from build123d import *

# Parameters (mm, degrees)
SKETCH_1_R      = 11
EXTRUDE_1_DEPTH = 7
SKETCH_2_R      = 6
EXTRUDE_2_DEPTH = 3
FILLET_1_R      = 2
THREAD_1_PITCH  = 1
SKETCH_9_W      = 0.25
SKETCH_9_H      = 0.05


with BuildPart() as part:
    # Sketch 1 → 凸台-拉伸1 (new body)
    with BuildSketch(Plane(origin=(0, 0, 0), x_dir=(1, 0, 0), z_dir=(0, 1, 0))):
        with Locations(Location((0, 0, 0), (0, 0, 270))):
            Circle(SKETCH_1_R)
    extrude(amount=EXTRUDE_1_DEPTH)

    # 草图2 → 凸台-拉伸2 (add)
    with BuildSketch(Plane(origin=(0, 7, 0), x_dir=(1, 0, 0), z_dir=(0, 1, 0))):
        with Locations(Location((0, 0, 0), (0, 0, 270))):
            Circle(SKETCH_2_R)
    extrude(amount=EXTRUDE_2_DEPTH)

    # 圆角1
    fillet_1_edges = [part.edges().sort_by_distance(p)[0] for p in [
        (0, 0, -11),
    ]]
    fillet(fillet_1_edges, radius=FILLET_1_R)

    # 螺纹线1: the profile of Sketch 1 2 profile screwed along a right-hand helix of 3 turns, 8 arcs to a turn; built about Z, then put on its axis
    thread_1_z = Axis((0, 0, 0), (0, 0, 1))
    thread_1_corners = [(5.9997, 0, -0.000173205), (6.541265875, 0, 0.312499999), (6.541265875, 0, 0.437499999), (5.9997, 0, 0.750173202)]
    with BuildLine(mode=Mode.PRIVATE) as thread_1_profile:
        Line(thread_1_corners[0], thread_1_corners[1])
        Line(thread_1_corners[1], thread_1_corners[2])
        Line(thread_1_corners[2], thread_1_corners[3])
        Line(thread_1_corners[3], thread_1_corners[0])
    thread_1_cap = Face(thread_1_profile.wire())
    thread_1_turn_angles = [0, 22.5, 45, 67.5, 90, 112.5, 135, 157.5, 180, 202.5, 225, 247.5, 270, 292.5, 315, 337.5, 360]
    thread_1_turn_weights = [1, 0.9238795325112867, 1, 0.9238795325112867, 1, 0.9238795325112867, 1, 0.9238795325112867, 1, 0.9238795325112867, 1, 0.9238795325112867, 1, 0.9238795325112867, 1, 0.9238795325112867, 1]
    thread_1_turn_rails = [Edge.make_bspline([Vector(p[0], p[1], 0).rotate(thread_1_z, thread_1_turn_angles[k]) / thread_1_turn_weights[k] + Vector(0, 0, p[2] + THREAD_1_PITCH * thread_1_turn_angles[k] / 360) for k in range(17)], [0, 0, 0, 1, 1, 2, 2, 3, 3, 4, 4, 5, 5, 6, 6, 7, 7, 8, 8, 8], 2, thread_1_turn_weights) for p in thread_1_corners]
    thread_1_turn_sides = [Face.make_surface_from_curves(thread_1_turn_rails[p[0]], thread_1_turn_rails[p[1]]) for p in [(0, 1), (1, 2), (2, 3), (3, 0)]]
    thread_1 = Plane(origin=(0, 10, 0), x_dir=(-1, 0, 0), z_dir=(0, -1, 0)) * Solid(Shell([*[p.moved(Location((0, 0, THREAD_1_PITCH * i))) for i in range(3) for p in thread_1_turn_sides], thread_1_cap, thread_1_cap.rotate(thread_1_z, 1080).moved(Location((0, 0, THREAD_1_PITCH * 1080 / 360)))]))
    add(thread_1)

    # 草图7 → 旋转1 (revolve)
    with BuildSketch(Plane.XY):
        Polygon((0, 10), (-9.5, 10), (-9.5, 10.3), (-9.089054213, 10.632548824), (-8.75, 10.5), (0, 10.5), align=None)
    revolve(axis=Axis((0, 10.5, 0), (0, -1, 0)))

    # 草图9 → 切除-旋转1 (revolve, cut)
    with BuildSketch(Plane.XY, mode=Mode.PRIVATE) as cut_revolve_1_sk:
        with Locations((-8.625, 10.475)):
            Rectangle(SKETCH_9_W, SKETCH_9_H)
    revolve(cut_revolve_1_sk.sketch.rotate(Axis((0, -0.995458227, 0), (0, 1, 0)), 270), axis=Axis((0, -0.995458227, 0), (0, 1, 0)), mode=Mode.SUBTRACT)


solid = part.part
Verification items for the finished model (mm, model axes). A direction names the side the tool comes from. Round coordinates to 2 decimals unless told otherwise and drop trailing zeros. Loops run counter-clockwise (first coordinate to the right, second up) from the corner with the lowest first, then second, coordinate; pieces in that order, holes last. Notation, with made-up numbers: (40, 71.25) - (76, 71.25) arc R35 cw to (76, 110.25) - close; hole circle Ø9 at (68.25, -19). An arc over 180 degrees is marked (long way). Use a Markdown table: item, result. Add a question column.
1. Gauge pin test, flat ends, axial feed: pin 1 (4 mm diameter, centred on y = 5, z = 7, fed in from -X); pin 2 (0.6 mm diameter, centred on x = -6.5, y = 9.5, fed in from +Z); pin 3 (4 mm diameter, centred on x = 3, y = 1.5, fed in from -Z). Record the tip position at first contact, or that the pin passes through.
2. Section check A-A, the plane y = 6.25. Record the boundary of the cut face in (x, z), plus the area to 3 significant figures.
3. Release check for a two-part mould opening along Z. For faces 4 (the face through (0, 10.5, 0)), 5 (the face through (-5, 7, 5)), 6 (the face through (-10.74, 4.46, -2.38)) record: released by +Z, released by -Z, zero draft, split by the parting line, or undercut.
4. Section check B-B, the plane y = 1.25. Record the boundary of the cut face in (x, z).
5. Access from +Z, -Z, +X, -X, +Y, -Y to the whole of each face (thin tool, end or side, straight path). Record for faces 1 (the face through (0, 0, 0)), 2 (the face through (-4.38, 10.15, 8.43)), 3 (the face through (-0.1, 10, 6.2)).
6. Thickness scan on probe 1 along Y at (x, z) = (5.25, 2.25); probe 2 along Y at (x, z) = (-7.75, 3); probe 3 along Y at (x, z) = (3.75, 5). Record the ranges inside material, lowest first. Write a range as [from, to].
Checks:
| question | item | result |
|---|---|---|
| 1 | pin 1 | stops at x = -9.8 |
| 1 | pin 2 | stops at z = 0 |
| 1 | pin 3 | stops at z = -10.95 |
| 2 | outline | circle Ø22 at (0, 0) |
| 2 | area | 380 mm^2 |
| 3 | face 4 | undercut |
| 3 | face 5 | zero draft |
| 3 | face 6 | split by the parting line |
| 4 | outline | circle Ø21.71 at (0, 0) |
| 5 | face 1 | +Z, -Z, +X, -X, -Y |
| 5 | face 2 | +Y |
| 5 | face 3 | none |
| 6 | probe 1 | y = [0, 10.5] |
| 6 | probe 2 | y = [0, 7], [10, 10.5] |
| 6 | probe 3 | y = [0, 7.21], [7.75, 8.21], [8.75, 9.21], [10, 10.5] |
